```python
from build123d import *

# Parameters (mm, degrees)
ESTRUSIONE_ESTRUSIONE1_DEPTH = 4
SCHIZZO2_W                   = 15
SCHIZZO2_H                   = 3
ESTRUSIONE_ESTRUSIONE2_DEPTH = 21


with BuildPart() as part:
    # Schizzo1 → Estrusione-Estrusione1 (new body)
    with BuildSketch(Plane.XY):
        with BuildLine():
            Line((0, 19.9), (0, 0))
            Line((0, 0), (15, 0))
            Line((15, 0), (15, 3.25))
            Line((15, 3.25), (9, 3.25))
            ThreePointArc((9, 3.25), (7.25, 5), (9, 6.75))
            Line((9, 6.75), (15, 6.75))
            Line((15, 6.75), (15, 13.15))
            Line((15, 13.15), (9, 13.15))
            ThreePointArc((9, 13.15), (7.25, 14.9), (9, 16.65))
            Line((9, 16.65), (15, 16.65))
            Line((15, 16.65), (15, 19.9))
            Line((15, 19.9), (0, 19.9))
        make_face()
    extrude(amount=ESTRUSIONE_ESTRUSIONE1_DEPTH)

    # Schizzo2 → Estrusione-Estrusione2 (add)
    with BuildSketch(Plane(origin=(0, 0, 0), x_dir=(-1, 0, 0), z_dir=(0, 0, -1))):
        with Locations((-7.5, 1.5)):
            Rectangle(SCHIZZO2_W, SCHIZZO2_H)
    extrude(amount=ESTRUSIONE_ESTRUSIONE2_DEPTH)


solid = part.part
```
Read the model definition and answer for the solid it produces. Units are mm, in the model's axes. A direction names the side the tool comes from. Coordinates: 2 decimals unless noted, no trailing zeros. Write each loop counter-clockwise with the first axis right and the second up, starting at its lowest first coordinate (ties: lowest second). Pieces come first, ordered by that corner, then holes. Notation, with made-up numbers: (50.5, 12.25) -> (80.5, 12.25) arc R28 ccw to (80.5, 44.25) -> close; hole circle Ø10 at (49.25, -26.5). An arc over 180 degrees is marked (long way). Return JSON: item names as keys, results as strings.
1. A tool of negligible diameter and unlimited length cuts with its end or side. For faces 1 (the face through (12, 13.15, 2)), 2 (the face through (7, 10, 4)), 3 (the face through (8, 3, -10)), from which of +Z, -Z, +X, -X, +Y, -Y can it reach the whole face along a straight path? Write none if from no direction.
Found:
{"face 1": "+Z, -Z, +X", "face 2": "+Z, +X, -X, +Y, -Y", "face 3": "-Z, +X, -X, +Y"}
2. Each of these flat-tipped pins is pushed along its axis until it touches: P1, Ø1.5, axis at x = 6, z = -3, coming from the -Y side; P2, Ø4.5, axis at x = 9.5, y = 15, coming from the -Z side; P3, Ø6, axis at x = 3, z = -10.5, coming from the +Y side; P4, Ø8, axis at y = 9, z = -10.5, coming from the +X side. Where does it stop, or does it pass through?
Found:
{"P1": "y = 0", "P2": "z = 0", "P3": "y = 3", "P4": "through"}
3. Determine the mould class of faces 4 (the face through (8, 19.9, 2)), 5 (the face through (12, 16.65, 2)), 6 (the face through (15, 2, -8)) for opening direction Y: pulls with the +Y half, pulls with the -Y half, needs draft (parallel to the pull), parting line crosses it, or undercut.
Found:
{"face 4": "pulls with the +Y half", "face 5": "undercut", "face 6": "needs draft"}
4. A cutting plane is placed at A-A (x = 11). Determine the outline of the cut face in (y, z), and give its area (3 significant figures).
Found:
{"outline": "(0, -21) -> (3, -21) -> (3, 0) -> (3.25, 0) -> (3.25, 4) -> (0, 4) -> close; (6.75, 0) -> (13.15, 0) -> (13.15, 4) -> (6.75, 4) -> close; (16.65, 0) -> (19.9, 0) -> (19.9, 4) -> (16.65, 4) -> close", "area": "115 mm2"}
5. Find the intervals of material crossed by line 1 along Y through (x, z) = (11.5, 1); line 2 along Z through (x, y) = (14, 12.75); line 3 along Y through (x, z) = (9.25, -1.5), in increasing order. Write a range as from..to.
Found:
{"line 1": "0..3.25, 6.75..13.15, 16.65..19.9", "line 2": "0..4", "line 3": "0..3"}
6. A cutting plane is placed at C-C (z = -12.5). Determine the outline of the cut face in (x, y).
Found:
{"outline": "(0, 0) -> (15, 0) -> (15, 3) -> (0, 3) -> close"}
7. A cutting plane is placed at D-D (x = 4). Determine the outline of the cut face in (y, z), and give its area (3 significant figures).
Found:
{"outline": "(0, -21) -> (3, -21) -> (3, 0) -> (19.9, 0) -> (19.9, 4) -> (0, 4) -> close", "area": "143 mm2"}
8. A cutting plane is placed at B-B (y = 14.9). Determine the outline of the cut face in (x, z), and give its area (3 significant figures).
Found:
{"outline": "(0, 0) -> (7.25, 0) -> (7.25, 4) -> (0, 4) -> close", "area": "29.0 mm2"}
